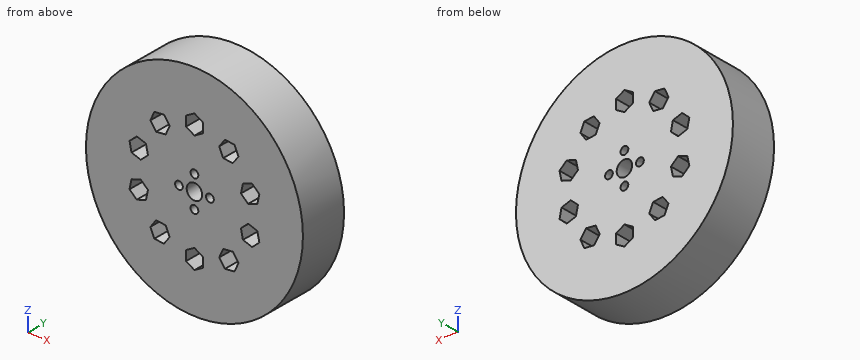
from build123d import *

# Parameters (mm, degrees)
F0_R     = 56
F0_R_2   = 21
F2_DEPTH = 12.5
F3_DEPTH = 25
F0_R_3   = 16
F0_R_4   = 2
F0_R_5   = 4
F4_DEPTH = 12.5


with BuildPart() as f2:
    # F0 (on Front) → F2 (new body, symmetric)
    with BuildSketch(Plane.XZ):
        with Locations((-66, 0)):
            Circle(F0_R)
        with Locations((-66, 0)):
            Circle(F0_R_2, mode=Mode.SUBTRACT)
    extrude(amount=F2_DEPTH, both=True)

    # F1 (on Front) → F3 (cut, symmetric)
    with BuildSketch(Plane.XZ):
        Polygon((-91.035729, 12.687567), (-95.791012, 14.232651), (-99.506736, 10.886998), (-98.467177, 5.99626), (-93.711895, 4.451175), (-89.996171, 7.796829), align=None)
        Polygon((-78.796766, 24.980089), (-81.735692, 29.025174), (-86.708302, 28.502532), (-88.741985, 23.934805), (-85.803059, 19.88972), (-80.830449, 20.412362), align=None)
        Polygon((-66, 25.231067), (-61.669873, 27.731067), (-61.669873, 32.731067), (-66, 35.231067), (-70.330127, 32.731067), (-70.330127, 27.731067), align=None)
        Polygon((-46.196941, 19.88972), (-43.258015, 23.934805), (-45.291698, 28.502532), (-50.264308, 29.025174), (-53.203234, 24.980089), (-51.169551, 20.412362), align=None)
        Polygon((-38.288105, 4.451175), (-33.532823, 5.99626), (-32.493264, 10.886998), (-36.208988, 14.232651), (-40.964271, 12.687567), (-42.003829, 7.796829), align=None)
        Polygon((-40.964271, -12.687567), (-36.208988, -14.232651), (-32.493264, -10.886998), (-33.532823, -5.99626), (-38.288105, -4.451175), (-42.003829, -7.796829), align=None)
        Polygon((-53.203234, -24.980089), (-50.264308, -29.025174), (-45.291698, -28.502532), (-43.258015, -23.934805), (-46.196941, -19.88972), (-51.169551, -20.412362), align=None)
        Polygon((-70.330127, -27.731067), (-70.330127, -32.731067), (-66, -35.231067), (-61.669873, -32.731067), (-61.669873, -27.731067), (-66, -25.231067), align=None)
        Polygon((-85.803059, -19.88972), (-88.741985, -23.934805), (-86.708302, -28.502532), (-81.735692, -29.025174), (-78.796766, -24.980089), (-80.830449, -20.412362), align=None)
        Polygon((-93.711895, -4.451175), (-98.467177, -5.99626), (-99.506736, -10.886998), (-95.791012, -14.232651), (-91.035729, -12.687567), (-89.996171, -7.796829), align=None)
    extrude(amount=F3_DEPTH, both=True, mode=Mode.SUBTRACT)

    # F0 (on Front) → F4 (join, symmetric)
    with BuildSketch(Plane.XZ):
        with Locations((-66, 0)):
            Circle(F0_R_2)
        with Locations((-66, 0)):
            Circle(F0_R_3, mode=Mode.SUBTRACT)
        with Locations((-66, 0)):
            Circle(F0_R_3)
        with Locations((-66, -8)):
            Circle(F0_R_4, mode=Mode.SUBTRACT)
        with Locations((-74, 0)):
            Circle(F0_R_4, mode=Mode.SUBTRACT)
        with Locations((-66, 0)):
            Circle(F0_R_5, mode=Mode.SUBTRACT)
        with Locations((-66, 8)):
            Circle(F0_R_4, mode=Mode.SUBTRACT)
        with Locations((-58, 0)):
            Circle(F0_R_4, mode=Mode.SUBTRACT)
    extrude(amount=F4_DEPTH, both=True)


solid = f2.part
Source: CAD feature listing. Evaluate the final solid. Frame: model axes, mm. Round coordinates to 2 decimals unless told otherwise and drop trailing zeros. Loops run counter-clockwise (first coordinate to the right, second up) from the corner with the lowest first, then second, coordinate; pieces in that order, holes last. Notation, with made-up numbers: M 89,59 L 96,59 A22 ccw 96,82 Z; hole C -37,6.25 d10. An arc over 180 degrees is marked long. Answer as CSV lines item,"result".
Q1. Cut plane B-B (y = -3.75). Count the separate pieces of the cut face and the enclosed holes in it, plus the area to 3 significant figures.
Verdict:
separate pieces,"1"
enclosed holes,"15"
area,"9,100 mm^2"
Q2. Contact query for flat-ended pins moving along their axis: pin 1 (4 mm diameter, centred on y = 5, z = 29.5, fed in from +X); pin 2 (12 mm diameter, centred on y = -4, z = -31.5, fed in from -X); pin 3 (12 mm diameter, centred on x = -65.5, y = -1, fed in from -Z). Output: stop coordinate, or through.
Verdict:
pin 1,"stops at x = -17.22"
pin 2,"stops at x = -115.86"
pin 3,"stops at z = -56"
Q3. Cut plane C-C (z = 17). Return the cut outline in (x, y).
Verdict:
outline,"M -119.36,-12.5 L -12.64,-12.5 L -12.64,12.5 L -119.36,12.5 Z"
Q4. Cut plane D-D (x = -20). Return the cut outline in (y, z).
Verdict:
outline,"M -12.5,-31.94 L 12.5,-31.94 L 12.5,31.94 L -12.5,31.94 Z"
Q5. Line query: line 1 along Z through (x, y) = (-66, -5.5); line 2 along Z through (x, y) = (-49.5, 4); line 3 along Z through (x, y) = (-40, -6.5). Output: solid intervals per line, ascending.
Verdict:
line 1,"z = -56 to -35.23, -25.23 to -10, -6 to -4, 4 to 6, 10 to 25.23, 35.23 to 56"
line 2,"z = -53.51 to -28.94, -20.24 to 20.24, 28.94 to 53.51"
line 3,"z = -49.6 to -13, -5.99 to 5.99, 13 to 49.6"
Q6. Cut plane A-A (x = -74). Return the cut outline in (y, z).
Verdict:
outline,"M -12.5,-55.43 L 12.5,-55.43 L 12.5,-2 L -12.5,-2 Z; M -12.5,2 L 12.5,2 L 12.5,55.43 L -12.5,55.43 Z"
